from build123d import *

# Parameters (mm, degrees)
SKETCH1_W           = 47.8
SKETCH1_H           = 40.6
BOSS_EXTRUDE1_DEPTH = 25.7
SKETCH2_W           = 41.8
SKETCH2_H           = 34.6
CUT_EXTRUDE1_DEPTH  = 23.2
FILLET1_R           = 2
SKETCH3_W           = 25
SKETCH3_H           = 25
CUT_EXTRUDE2_DEPTH  = 40.006922463
CUT_EXTRUDE3_START  = 22.2
SKETCH4_W           = 47
SKETCH4_H           = 37
CUT_EXTRUDE3_DEPTH  = 2.3
SKETCH6_W           = 37
SKETCH6_H           = 3.5
CUT_EXTRUDE4_DEPTH  = 4
SKETCH7_W           = 15
SKETCH7_H           = 13
CUT_EXTRUDE5_DEPTH  = 4
FILLET2_R           = 2


with BuildPart() as part:
    # Sketch1 → Boss-Extrude1 (new body)
    with BuildSketch(Plane(origin=(0, 0, 0), x_dir=(1, 0, 0), z_dir=(0, 1, 0))):
        Rectangle(SKETCH1_W, SKETCH1_H)
    extrude(amount=BOSS_EXTRUDE1_DEPTH)

    # Sketch2 → Cut-Extrude1 (cut)
    with BuildSketch(Plane(origin=(0, 25.7, 0), x_dir=(1, 0, 0), z_dir=(0, 1, 0))):
        Rectangle(SKETCH2_W, SKETCH2_H)
    extrude(amount=-CUT_EXTRUDE1_DEPTH, mode=Mode.SUBTRACT)

    # Fillet1
    fillet1_edges = [part.edges().sort_by_distance(p)[0] for p in [
        (23.9, 12.85, 20.3),
        (-23.9, 12.85, 20.3),
        (-23.9, 12.85, -20.3),
        (23.9, 12.85, -20.3),
    ]]
    fillet(fillet1_edges, radius=FILLET1_R)

    # Sketch3 → Cut-Extrude2 (cut, through all)
    with BuildSketch(Plane(origin=(0, 2.5, 0), x_dir=(1, 0, 0), z_dir=(0, 1, 0))):
        with Locations((5.75, 0)):
            Rectangle(SKETCH3_W, SKETCH3_H)
    extrude(amount=-CUT_EXTRUDE2_DEPTH, mode=Mode.SUBTRACT)

    # Sketch4 → Cut-Extrude3 (cut)
    with BuildSketch(Plane(origin=(0, 0, 0), x_dir=(1, 0, 0), z_dir=(0, 1, 0)).offset(CUT_EXTRUDE3_START)):
        with Locations((-1.4, 0)):
            Rectangle(SKETCH4_W, SKETCH4_H)
    extrude(amount=CUT_EXTRUDE3_DEPTH, mode=Mode.SUBTRACT)

    # Sketch6 → Cut-Extrude4 (cut)
    with BuildSketch(Plane.ZY.offset(23.9)):
        with Locations((0, 25.7)):
            Rectangle(SKETCH6_W, SKETCH6_H)
    extrude(amount=-CUT_EXTRUDE4_DEPTH, mode=Mode.SUBTRACT)

    # Sketch7 → Cut-Extrude5 (cut)
    with BuildSketch(Plane.ZY.offset(23.9)):
        with Locations((0, 22.2)):
            Rectangle(SKETCH7_W, SKETCH7_H)
    extrude(amount=-CUT_EXTRUDE5_DEPTH, mode=Mode.SUBTRACT)

    # Fillet2
    fillet2_edges = [part.edges().sort_by_distance(p)[0] for p in [
        (-22.4, 15.7, 7.5),
        (-22.4, 15.7, -7.5),
    ]]
    fillet(fillet2_edges, radius=FILLET2_R)


solid = part.part
Geometry check sheet. Reference: the model listing, model coordinates, mm. A direction names the side the tool comes from. Give positions to 0.01 mm unless a question says otherwise; leave off trailing zeros. Order: outer loops, then holes, each group sorted by start corner. A loop starts at its lowest first (then second) coordinate and runs counter-clockwise, first axis right, second up. Notation, with made-up numbers: (-24, 29.5) - (22, 29.5) arc R24 cw to (22, 44.5) - close; hole circle Ø7 at (62, 69.25). An arc over 180 degrees is marked (long way). Answer as a JSON object with one key per item and string values.
(1) Draft check along X on faces 1 (the cylindrical face through (-23.33, 13.03, 19.7)), 2 (the flat face through (23.9, 13, 0)), 3 (the flat face through (6, 1, 12.5)). Enter one of: released by +X, released by -X, zero draft, split by the parting line, or undercut.
Report:
{"face 1": "released by -X", "face 2": "released by +X", "face 3": "undercut"}
(2) Depth check by flat-ended pin: pin 1 Ø1.3 at (y, z) = (25.5, 1) entering from -X; pin 2 Ø1.3 at (y, z) = (25, -18) entering from -X; pin 3 Ø10 at (x, z) = (-16.5, -6.5) entering from +Y. Enter the tip coordinate at first touch or a pass-through.
Report:
{"pin 1": "x = 20.9", "pin 2": "x = -23.89", "pin 3": "y = 22.2"}
(3) Cross-section at D-D (z = -14). Record the cut outline in (x, y), then the cut area to 3 significant figures.
Report:
{"outline": "(-23.9, 0) - (23.9, 0) - (23.9, 25.7) - (20.9, 25.7) - (20.9, 24.5) - (22.1, 24.5) - (22.1, 22.2) - (20.9, 22.2) - (20.9, 2.5) - (-20.9, 2.5) - (-20.9, 22.2) - (-23.9, 22.2) - close", "area": "245 mm^2"}
(4) Tool access check on faces 4 (the flat face through (0, 25, -17.3)), 5 (the flat face through (-1, 22.2, -18)), 6 (the flat face through (6, 1, -12.5)). Record the directions out of +Z, -Z, +X, -X, +Y, -Y that give a thin tool (end or side, any length) a straight path to the whole face; none if there is none.
Report:
{"face 4": "-X, +Y", "face 5": "-X", "face 6": "+Y, -Y"}
(5) Cross-section at B-B (x = 14.5). Record the cut outline in (y, z).
Report:
{"outline": "(0, -20.3) - (25.7, -20.3) - (25.7, -17.3) - (24.5, -17.3) - (24.5, -18.5) - (22.2, -18.5) - (22.2, -17.3) - (2.5, -17.3) - (2.5, -12.5) - (0, -12.5) - close; (0, 12.5) - (2.5, 12.5) - (2.5, 17.3) - (22.2, 17.3) - (22.2, 18.5) - (24.5, 18.5) - (24.5, 17.3) - (25.7, 17.3) - (25.7, 20.3) - (0, 20.3) - close"}
(6) Cross-section at A-A (z = 10). Record the cut outline in (x, y).
Report:
{"outline": "(-23.9, 0) - (-6.75, 0) - (-6.75, 2.5) - (-20.9, 2.5) - (-20.9, 22.2) - (-23.9, 22.2) - close; (18.25, 0) - (23.9, 0) - (23.9, 25.7) - (20.9, 25.7) - (20.9, 24.5) - (22.1, 24.5) - (22.1, 22.2) - (20.9, 22.2) - (20.9, 2.5) - (18.25, 2.5) - close"}
(7) Material ranges on line 1 (X direction, y = 12.25, z = 6.5); line 2 (Z direction, x = 6, y = 5); line 3 (Y direction, x = 12, z = 18), recorded low to high.
Report:
{"line 1": "-23.9 to -20.9, 20.9 to 23.9", "line 2": "-20.3 to -17.3, 17.3 to 20.3", "line 3": "0 to 22.2, 24.5 to 25.7"}
(8) Cross-section at C-C (y = 14). Record the cut outline in (x, z), then the cut area to 3 significant figures.
Report:
{"outline": "(-23.9, -18.3) arc R2 ccw to (-21.9, -20.3) - (21.9, -20.3) arc R2 ccw to (23.9, -18.3) - (23.9, 18.3) arc R2 ccw to (21.9, 20.3) - (-21.9, 20.3) arc R2 ccw to (-23.9, 18.3) - close; hole (-20.9, -17.3) - (20.9, -17.3) - (20.9, 17.3) - (-20.9, 17.3) - close", "area": "491 mm^2"}
